from build123d import *

# Parameters (mm, degrees)
SKETCH1_W          = 10
SKETCH1_H          = 37
SKETCH2_R          = 8.5
CUT_EXTRUDE1_DEPTH = 181
FILLET1_R          = 1
CHAMFER1_SIZE      = 1


with BuildPart() as part:
    # Sketch1 → Revolve1 (revolve)
    with BuildSketch(Plane.XY, mode=Mode.PRIVATE) as revolve1_sk:
        Polygon((27.5, 9.5), (27.5, 0), (120, 0), (120, 60), (90, 60), (90, 56), (27.5, 56), (27.5, 46.5), (37.5, 46.5), (37.5, 9.5), align=None)
        with Locations((32.5, 28)):
            Rectangle(SKETCH1_W, SKETCH1_H)
        with Locations((22.5, 28)):
            Rectangle(SKETCH1_W, SKETCH1_H)
    revolve(revolve1_sk.sketch.rotate(Axis((0, 0, 0), (0, 1, 0)), 90), axis=Axis((0, 0, 0), (0, 1, 0)))

    # Sketch2 → Cut-Extrude1 (cut, through all)
    with BuildSketch(Plane(origin=(0, 60, 0), x_dir=(1, 0, 0), z_dir=(0, 1, 0))):
        with Locations(Location((-74.953318805, 74.953318805, 0), (0, 0, 270))):
            Circle(SKETCH2_R)
        with Locations(Location((74.953318805, 74.953318805, 0), (0, 0, 270))):
            Circle(SKETCH2_R)
        with Locations(Location((74.953318805, -74.953318805, 0), (0, 0, 270))):
            Circle(SKETCH2_R)
        with Locations(Location((-74.953318805, -74.953318805, 0), (0, 0, 270))):
            Circle(SKETCH2_R)
    extrude(amount=-CUT_EXTRUDE1_DEPTH, mode=Mode.SUBTRACT)

    # Fillet1
    fillet1_edges = [part.edges().sort_by_distance(p)[0] for p in [
        (0, 56, 27.5),
        (0, 60, 120),
    ]]
    fillet(fillet1_edges, radius=FILLET1_R)

    # Chamfer1
    chamfer1_edges = [part.edges().sort_by_distance(p)[0] for p in [
        (0, 9.5, 17.5),
        (0, 46.5, 17.5),
    ]]
    chamfer(chamfer1_edges, length=CHAMFER1_SIZE)


solid = part.part
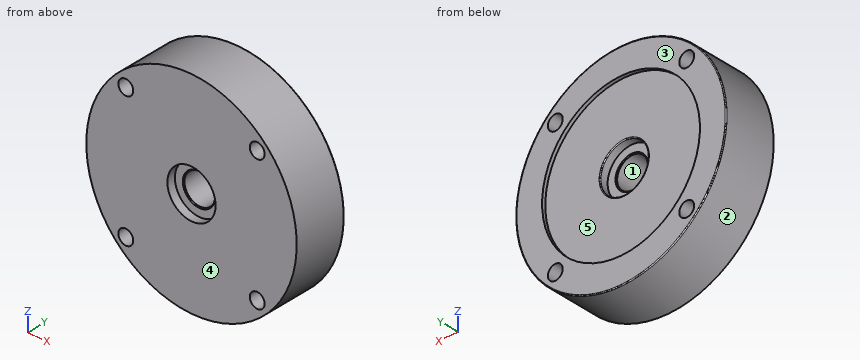
Design review of the part built by this model. Coordinates are the model's own, in mm. Face numbers are marked on the shaded views. A direction names the side the tool comes from. Round coordinates to 2 decimals unless told otherwise and drop trailing zeros. Write each loop counter-clockwise with the first axis right and the second up, starting at its lowest first coordinate (ties: lowest second). Pieces come first, ordered by that corner, then holes. Notation, with made-up numbers: M 12.5,-34.75 L 48.5,-34.75 A28 cw 48.5,-6.75 Z; hole C 7.25,17.25 d7. An arc over 180 degrees is marked long. One line per item, written item: value. Start each with the question number.
1. Take a section at C-C on y = 40. State the section outline as (x, z) points, then the cut area to 3 significant figures.
2. To check wall thickness, follow probe 1 along X at (y, z) = (33, 0); probe 2 along X at (y, z) = (50.75, 0); probe 3 along Z at (x, y) = (74, 43). State the ranges of each line that lie inside material, in increasing order. Write a range as from..to.
3. Take a section at B-B on z = 0. State the section outline as (x, y) points, then the cut area to 3 significant figures.
4. For the marked faces 4 and 5, list the 3-axis set-ups (+Z, -Z, +X, -X, +Y, -Y) from which the entire face can be reached by the end or side of a thin tool; tool diameter is ignored.
5. Clearance check with flat-ended pins moving along their axes: P1, Ø10, axis at x = 55, y = 21.5, coming from the +Z side; P2, Ø5, axis at y = 17.5, z = -28, coming from the +X side; P3, Ø3, axis at x = -41, z = 56, coming from the +Y side; P4, Ø15.5, axis at x = 74.95, z = -74.95, coming from the +Y side. State where each tip first meets the part, or that it passes through.
6. Take a section at A-A on x = 0. State the section outline as (y, z) points.
7. Draft analysis for pull direction X (two halves, no side actions). For the marked faces 1, 2 and 3, state which applies: pulls with the +X half, pulls with the -X half, needs draft (parallel to the pull), parting line crosses it, or undercut.
Computed:
1. outline: C 0,0 d240; hole C -74.95,-74.95 d17; hole C -74.95,74.95 d17; hole C 0,0 d35; hole C 74.95,-74.95 d17; hole C 74.95,74.95 d17
1. area: 43,400 mm²
2. probe 1: x = -120..-17.5, 17.5..120
2. probe 2: x = -120..-27.5, 27.5..120
2. probe 3: z = -94.47..-83.4, -66.51..66.51, 83.4..94.47
3. outline: M -120,0 L -27.5,0 L -27.5,9.5 L -18.5,9.5 L -17.5,10.5 L -17.5,45.5 L -18.5,46.5 L -27.5,46.5 L -27.5,55 A1 ccw -28.5,56 L -90,56 L -90,60 L -119,60 A1 ccw -120,59 Z; M 17.5,10.5 L 18.5,9.5 L 27.5,9.5 L 27.5,0 L 120,0 L 120,59 A1 ccw 119,60 L 90,60 L 90,56 L 28.5,56 A1 ccw 27.5,55 L 27.5,46.5 L 18.5,46.5 L 17.5,45.5 Z
3. area: 11,300 mm²
4. face 4: +Z, -Z, +X, -X, -Y
4. face 5: +Y
5. P1: stops at z = 109.09
5. P2: stops at x = 117.26
5. P3: stops at y = 56
5. P4: passes through
6. outline: M 0,-120 L 59,-120 A1 ccw 60,-119 L 60,-90 L 56,-90 L 56,-28.5 A1 ccw 55,-27.5 L 46.5,-27.5 L 46.5,-18.5 L 45.5,-17.5 L 10.5,-17.5 L 9.5,-18.5 L 9.5,-27.5 L 0,-27.5 Z; M 0,27.5 L 9.5,27.5 L 9.5,18.5 L 10.5,17.5 L 45.5,17.5 L 46.5,18.5 L 46.5,27.5 L 55,27.5 A1 ccw 56,28.5 L 56,90 L 60,90 L 60,119 A1 ccw 59,120 L 0,120 Z
7. face 1: undercut
7. face 2: parting line crosses it
7. face 3: needs draft
